Study the drawing (mm; zero at the part's minimum x, y, z) and answer. Coordinates: 2 decimals unless noted, no trailing zeros. Loops run counter-clockwise (first coordinate to the right, second up) from the corner with the lowest first, then second, coordinate; pieces in that order, holes last. Notation, with made-up numbers: (-3.75, 42.25) - (49.25, 42.25) arc R20 cw to (49.25, 51.25) - close; hole circle Ø5 at (58.25, -23.5). An arc over 180 degrees is marked (long way). Use CSV: the item, a comma, the result in double quotes.
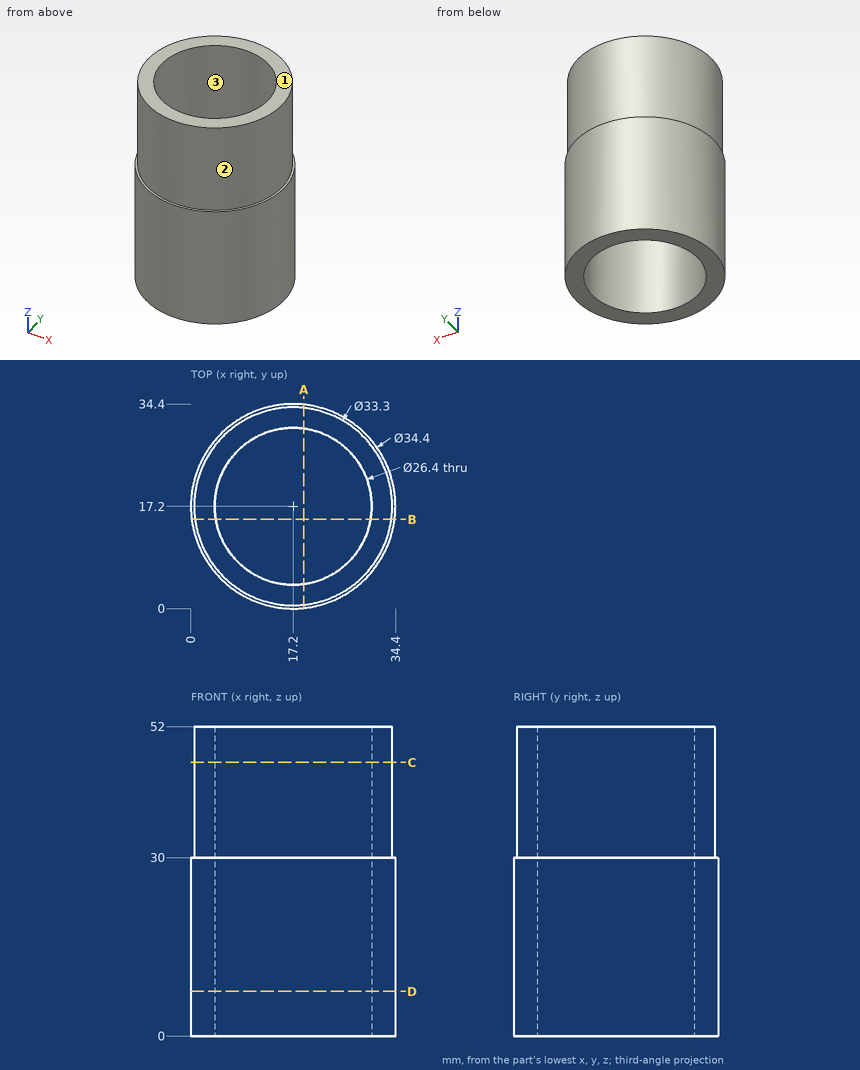
Q1. Given P1, Ø1, axis at y = 27.5, z = 22.5, coming from the +X side; P2, Ø8, axis at x = 6, z = 27, coming from the -Y side; P3, Ø1, axis at x = 25, z = 10, coming from the +Y side, each flat-ended and moving along its own axis, determine where each tip first touches the part or whether it passes through.
Reported:
P1,"stops at x = 31.34"
P2,"stops at y = 1.58"
P3,"stops at y = 32.77"
Q2. The part is cut by section B-B on y = 15. Determine the outline of the cut face in (x, z).
Reported:
outline,"(0.14, 0) - (4.18, 0) - (4.18, 52) - (0.7, 52) - (0.7, 30) - (0.14, 30) - close; (30.22, 0) - (34.26, 0) - (34.26, 30) - (33.7, 30) - (33.7, 52) - (30.22, 52) - close"
Q3. For a pull along Y with two mould halves and no side action, classify the marked faces 1, 2 and 3 as +Y half, -Y half, draft (parallel to the pull), parting line (faces both ways), or undercut.
Reported:
face 1,"draft"
face 2,"parting line"
face 3,"undercut"
Q4. Find the intervals of material crossed by probe 1 along Y at (x, z) = (17.2, 30.5); probe 2 along Y at (x, z) = (17, 14), in increasing order. Write a range as [from, to].
Reported:
probe 1,"y = [0.55, 4], [30.4, 33.85]"
probe 2,"y = [0, 4], [30.4, 34.4]"
Q5. The part is cut by section D-D on z = 7.5. Determine the outline of the cut face in (x, y), and give its area (3 significant figures).
Reported:
outline,"circle Ø34.4 at (17.2, 17.2); hole circle Ø26.4 at (17.2, 17.2)"
area,"382 mm²"
Q6. The part is cut by section A-A on x = 19. Determine the outline of the cut face in (y, z).
Reported:
outline,"(0.09, 0) - (4.12, 0) - (4.12, 52) - (0.65, 52) - (0.65, 30) - (0.09, 30) - close; (30.28, 0) - (34.31, 0) - (34.31, 30) - (33.75, 30) - (33.75, 52) - (30.28, 52) - close"
Q7. The part is cut by section C-C on z = 46. Determine the outline of the cut face in (x, y), and give its area (3 significant figures).
Reported:
outline,"circle Ø33.3 at (17.2, 17.2); hole circle Ø26.4 at (17.2, 17.2)"
area,"324 mm²"
